```python
from build123d import *

# Parameters (mm, degrees)
SKETCH1_W           = 27.94
SKETCH1_H           = 28.956
SKETCH1_W_2         = 6.35
SKETCH1_H_2         = 6.35
SKETCH1_W_3         = 1.7272
SKETCH1_H_3         = 2.032
BOSS_EXTRUDE1_DEPTH = 1.7272
SKETCH3_W           = 2.032
SKETCH3_H           = 1.7272
CUT_EXTRUDE1_DEPTH  = 1.7272
SKETCH4_R           = 4.572
SKETCH4_R_2         = 2.794
CUT_EXTRUDE4_DEPTH  = 1.7272


with BuildPart() as part:
    # Sketch1 → Boss-Extrude1 (new body)
    with BuildSketch(Plane(origin=(0, 0, 0), x_dir=(0, 0, -1), z_dir=(1, 0, 0))):
        with Locations((13.97, 14.478)):
            Rectangle(SKETCH1_W, SKETCH1_H)
        with Locations((8.89, 8.5598)):
            Rectangle(SKETCH1_W_2, SKETCH1_H_2, mode=Mode.SUBTRACT)
        with Locations((26.5684, 4.826)):
            Rectangle(SKETCH1_W_3, SKETCH1_H_3, mode=Mode.SUBTRACT)
        with Locations((26.5684, 27.178)):
            Rectangle(SKETCH1_W_3, SKETCH1_H_3, mode=Mode.SUBTRACT)
    extrude(amount=BOSS_EXTRUDE1_DEPTH)

    # Sketch3 → Cut-Extrude1 (cut)
    with BuildSketch(Plane(origin=(1.7272, 0, 0), x_dir=(0, 0, -1), z_dir=(1, 0, 0))):
        with Locations((3.6068, 1.50495)):
            Rectangle(SKETCH3_W, SKETCH3_H)
        with Locations((23.9268, 1.50495)):
            Rectangle(SKETCH3_W, SKETCH3_H)
    extrude(amount=-CUT_EXTRUDE1_DEPTH, mode=Mode.SUBTRACT)

    # Sketch4 → Cut-Extrude4 (cut)
    with BuildSketch(Plane(origin=(1.7272, 0, 0), x_dir=(0, 0, -1), z_dir=(1, 0, 0))):
        with BuildLine():
            ThreePointArc((9.569657679, 11.7348), (12.354864998, 13.273066118), (13.462, 16.256))
            ThreePointArc((13.462, 16.256), (10.193220511, 20.638328183), (5.06095, 18.754311449))
            ThreePointArc((5.06095, 18.754311449), (6.18714012, 17.724210084), (6.604, 16.256))
            ThreePointArc((6.604, 16.256), (6.18714012, 14.787789916), (5.06095, 13.757688551))
            ThreePointArc((5.06095, 13.757688551), (6.41914372, 12.409176213), (8.210342321, 11.7348))
            Line((8.210342321, 11.7348), (9.569657679, 11.7348))
        make_face()
        with Locations((8.89, 16.256)):
            Circle(SKETCH4_R)
        with Locations((3.81, 16.256)):
            Circle(SKETCH4_R_2)
    extrude(amount=-CUT_EXTRUDE4_DEPTH, mode=Mode.SUBTRACT)


solid = part.part
```
The listing builds one solid part. Answer for the finished solid, in the listing's coordinates (mm). A direction names the side the tool comes from. Give positions to 0.01 mm unless a question says otherwise; leave off trailing zeros. Order: outer loops, then holes, each group sorted by start corner. A loop starts at its lowest first (then second) coordinate and runs counter-clockwise, first axis right, second up. Notation, with made-up numbers: (75.5, 28.5) -> (114.5, 28.5) arc R25 cw to (114.5, 63.5) -> close; hole circle Ø3 at (-17, 20). An arc over 180 degrees is marked (long way). Answer as a JSON object with one key per item and string values. Group by question number.
Item 1: The part is cut by section A-A on z = -3.81. Write down the section's boundary in (x, y), and give its area (3 significant figures).
Item 2: The part is cut by section B-B on y = 7. Write down the section's boundary in (x, z) (3 decimals), and give its area (3 significant figures).
Item 3: Consider L1, parallel to Z at x = 1, y = 1; L2, parallel to Y at x = 0.5, z = -3.81; L3, parallel to Z at x = 0.6, y = 27.5. Determine where each line is inside the solid, lowest interval first. Write a range as from..to.
Item 4: The part is cut by section C-C on x = 0.45. Write down the section's boundary in (y, z) (3 decimals), and give its area (3 significant figures).
Item 5: Determine the mould class of faces 1 (the flat face through (1, 14, 0)), 2 (the flat face through (1, 28.956, -14)), 3 (the flat face through (1, 1, -4.623)) for opening direction Z: pulls with the +Z half, pulls with the -Z half, needs draft (parallel to the pull), parting line crosses it, or undercut.
Item 6: A tool of negligible diameter and unlimited length cuts with its end or side. For faces 4 (the flat face through (1, 0, -14)), 5 (the flat face through (1, 5, -25.705)), from which of +Z, -Z, +X, -X, +Y, -Y can it reach the whole face along a straight path? Write none if from no direction.
Item 7: The part is cut by section D-D on y = 14.5. Write down the section's boundary in (x, z).
Result set:
{
 "1": {"outline": "(0, 0) -> (1.73, 0) -> (1.73, 0.64) -> (0, 0.64) -> close; (0, 2.37) -> (1.73, 2.37) -> (1.73, 13.46) -> (0, 13.46) -> close; (0, 19.05) -> (1.73, 19.05) -> (1.73, 28.96) -> (0, 28.96) -> close", "area": "37.4 mm²"},
 "2": {"outline": "(0, -27.94) -> (1.727, -27.94) -> (1.727, -12.065) -> (0, -12.065) -> close; (0, -5.715) -> (1.727, -5.715) -> (1.727, 0) -> (0, 0) -> close", "area": "37.3 mm²"},
 "3": {"L1": "-27.94..-24.94, -22.91..-4.62, -2.59..0", "L2": "0..0.64, 2.37..13.46, 19.05..28.96", "L3": "-27.94..-27.43, -25.7..0"},
 "4": {"outline": "(0, -27.94) -> (28.956, -27.94) -> (28.956, 0) -> (0, 0) -> close; hole (0.641, -24.943) -> (2.369, -24.943) -> (2.369, -22.911) -> (0.641, -22.911) -> close; hole (0.641, -4.623) -> (2.369, -4.623) -> (2.369, -2.591) -> (0.641, -2.591) -> close; hole (3.81, -27.432) -> (5.842, -27.432) -> (5.842, -25.705) -> (3.81, -25.705) -> close; hole (5.385, -12.065) -> (11.735, -12.065) -> (11.735, -9.57) arc R4.572 ccw (long way) to (18.754, -5.061) arc R2.794 ccw (long way) to (13.758, -5.061) arc R4.572 ccw to (11.735, -8.21) -> (11.735, -5.715) -> (5.385, -5.715) -> close; hole (26.162, -27.432) -> (28.194, -27.432) -> (28.194, -25.705) -> (26.162, -25.705) -> close", "area": "673 mm²"},
 "5": {"face 1": "pulls with the +Z half", "face 2": "needs draft", "face 3": "undercut"},
 "6": {"face 4": "+Z, -Z, +X, -X, -Y", "face 5": "+X, -X"},
 "7": {"outline": "(0, -27.94) -> (1.73, -27.94) -> (1.73, -13.11) -> (0, -13.11) -> close; (0, -1.64) -> (1.73, -1.64) -> (1.73, 0) -> (0, 0) -> close"}
}
